Check sheet for the modelled part. Datum: model origin and axes. Units: mm. Face numbers are marked on the shaded views. Give positions to 0.01 mm unless a question says otherwise; leave off trailing zeros. Loops run counter-clockwise (first coordinate to the right, second up) from the corner with the lowest first, then second, coordinate; pieces in that order, holes last. Notation, with made-up numbers: M 0,-36.75 L 27,-36.75 A25 cw 27,-24.75 Z; hole C 59.25,11 d9. An arc over 180 degrees is marked long. Use one line per item in the form item = value.
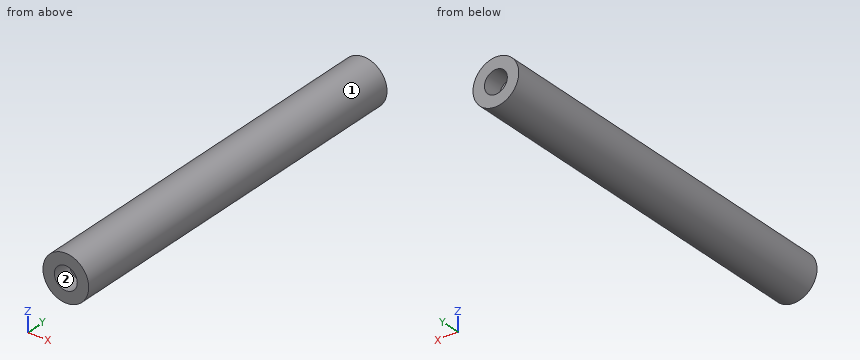
from build123d import *

# Parameters (mm, degrees)
SKETCH1_R           = 6
SKETCH1_R_2         = 1.5
BOSS_EXTRUDE1_DEPTH = 100
SKETCH2_R           = 3
CUT_EXTRUDE1_DEPTH  = 5
SKETCH3_R           = 3
CUT_EXTRUDE2_DEPTH  = 5


with BuildPart() as part:
    # Sketch1 → Boss-Extrude1 (new body)
    with BuildSketch(Plane(origin=(0, 0, 0), x_dir=(1, 0, 0), z_dir=(0, 1, 0))):
        Circle(SKETCH1_R)
        Circle(SKETCH1_R_2, mode=Mode.SUBTRACT)
    extrude(amount=BOSS_EXTRUDE1_DEPTH)

    # Sketch2 → Cut-Extrude1 (cut)
    with BuildSketch(Plane(origin=(0, 100, 0), x_dir=(1, 0, 0), z_dir=(0, 1, 0))):
        Circle(SKETCH2_R)
    extrude(amount=-CUT_EXTRUDE1_DEPTH, mode=Mode.SUBTRACT)

    # Sketch3 → Cut-Extrude2 (cut)
    with BuildSketch(Plane.XZ):
        Circle(SKETCH3_R)
    extrude(amount=-CUT_EXTRUDE2_DEPTH, mode=Mode.SUBTRACT)


solid = part.part
1) Section check A-A (z = 0). Record the cut outline in (x, y).
Evaluation:
outline = M -6,0 L -3,0 L -3,5 L -1.5,5 L -1.5,95 L -3,95 L -3,100 L -6,100 Z; M 1.5,5 L 3,5 L 3,0 L 6,0 L 6,100 L 3,100 L 3,95 L 1.5,95 Z
2) Release check for a two-part mould opening along X. For the marked faces 1 and 2 record: pulls with the +X half, pulls with the -X half, needs draft (parallel to the pull), parting line crosses it, or undercut.
Evaluation:
face_1 = parting line crosses it
face_2 = undercut
3) Scan lines: line 1 (Z direction, x = 0, y = 56.5); line 2 (Z direction, x = 0, y = 97.15). Record each from-to range of solid material in increasing order.
Evaluation:
line_1 = -6 to -1.5, 1.5 to 6
line_2 = -6 to -3, 3 to 6
4) Section check D-D (x = 4.5). Record the cut outline in (y, z).
Evaluation:
outline = M 0,-3.97 L 100,-3.97 L 100,3.97 L 0,3.97 Z
5) Section check B-B (x = 0). Record the cut outline in (y, z), then the cut area to 3 significant figures.
Evaluation:
outline = M 0,-6 L 100,-6 L 100,-3 L 95,-3 L 95,-1.5 L 5,-1.5 L 5,-3 L 0,-3 Z; M 0,3 L 5,3 L 5,1.5 L 95,1.5 L 95,3 L 100,3 L 100,6 L 0,6 Z
area = 870 mm^2
6) Depth check by flat-ended pin: pin 1 Ø3 at (x, y) = (2, 33) entering from -Z; pin 2 Ø1 at (x, y) = (3, 66.5) entering from +Z. Enter the tip coordinate at first touch or a pass-through.
Evaluation:
pin_1 = -5.98
pin_2 = 5.45
7) Section check C-C (y = 44). Record the cut outline in (x, z), then the cut area to 3 significant figures.
Evaluation:
outline = C 0,0 d12; hole C 0,0 d3
area = 106 mm^2
